The listing builds one solid part. Answer for the finished solid, in the listing's coordinates (mm). Face numbers are marked on the shaded views. A direction names the side the tool comes from. Round coordinates to 2 decimals unless told otherwise and drop trailing zeros. Order: outer loops, then holes, each group sorted by start corner. A loop starts at its lowest first (then second) coordinate and runs counter-clockwise, first axis right, second up. Notation, with made-up numbers: M 17,63 L 62,63 A17 cw 62,70 Z; hole C 74,59.25 d7. An arc over 180 degrees is marked long. Write item = value, one per line. Start each with the question number.
(1) A cutting plane is placed at C-C, the plane y = -41. Determine the outline of the cut face in (x, z).
(2) A cutting plane is placed at D-D, the plane x = -1. Determine the outline of the cut face in (y, z).
(3) For a pull along X with two mould halves and no side action, classify the marked faces 1, 2, 3 and 4 as released by +X, released by -X, zero draft, split by the parting line, or undercut.
(4) Straight lines are drawn through the part: probe 1 along X at (y, z) = (-48, 10.5); probe 2 along X at (y, z) = (-44, 1.5); probe 3 along Y at (x, z) = (19, 5). For each, find the intervals that lie inside material, in ascending order. Write a range as from..to.
(5) Which of the six approach directions +Z, -Z, +X, -X, +Y, -Y give full straight-line access (tool end or side, diameter ignored) to the marked faces 5, 6 and 7?
(6) Each of these flat-tipped pins is pushed along its axis until it touches: pin 1 (0.5 mm diameter, centred on y = -54.5, z = 10.5, fed in from -X); pin 2 (2.5 mm diameter, centred on x = -61.5, z = 6.5, fed in from +Y); pin 3 (6 mm diameter, centred on x = -56.5, z = 11, fed in from -Y). Where does it stop, or does it pass through?
(7) A cutting plane is placed at B-B, the plane x = -88. Determine the outline of the cut face in (y, z), and give its area (3 significant figures).
(8) A cutting plane is placed at A-A, the plane z = 9. Determine the outline of the cut face in (x, y).
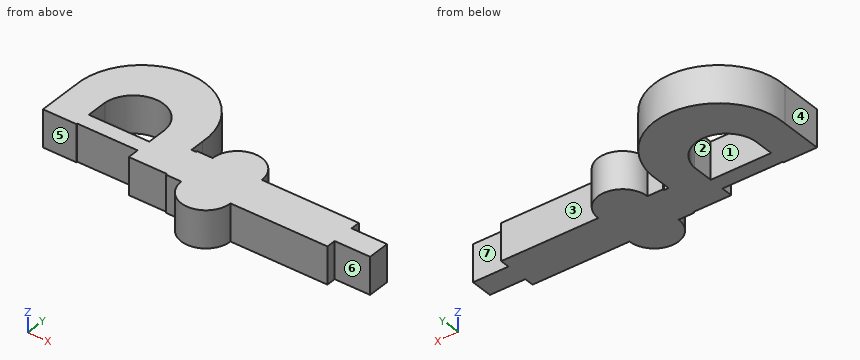
from build123d import *

# Parameters (mm, degrees)
F0_W     = 17
F0_H     = 10.514781
F1_DEPTH = 17.78


with BuildPart() as f1:
    # F0 (on Top) → F1 (new body)
    with BuildSketch(Plane.XY):
        with BuildLine():
            Line((-63.051145, -54.98954), (-63.051145, -48.261526))
            ThreePointArc((-63.051145, -48.261526), (-93.559145, -15.989189), (-124.067145, -48.261526))
            Line((-124.067145, -48.261526), (-124.067145, -54.989189))
            Line((-124.067145, -54.989189), (-124.067145, -56.005189))
            Line((-124.067145, -56.005189), (-124.067145, -68.254414))
            Line((-124.067145, -68.254414), (-108.051145, -68.254414))
            Line((-108.051145, -68.254414), (-108.051145, -67.754308))
            Line((-108.051145, -67.754308), (-108.051145, -60.490071))
            Line((-108.051145, -60.490071), (-108.051145, -56.005189))
            Line((-108.051145, -56.005189), (-108.051145, -54.989189))
            Line((-108.051145, -54.989189), (-108.051145, -50.514857))
            ThreePointArc((-108.051145, -50.514857), (-93.559145, -37.005189), (-79.067145, -50.514857))
            Line((-79.067145, -50.514857), (-79.067145, -54.98954))
            Line((-79.067145, -54.98954), (-63.051145, -54.98954))
        make_face()
        Polygon((-79.067145, -61.005189), (-79.067145, -60.490071), (-108.051145, -60.490071), (-108.051145, -67.754308), (-79.067145, -67.754308), align=None)
        Polygon((-60.801145, -54.98954), (-63.051145, -54.98954), (-79.067145, -54.98954), (-79.067145, -60.490071), (-79.067145, -61.005189), (-79.067145, -67.754308), (-79.067145, -73.254839), (-60.801145, -73.254839), align=None)
        Polygon((-60.801145, -54.364518), (-60.801145, -54.98954), (-60.801145, -73.254839), (-60.801145, -73.879861), (-53.390384, -73.879861), (-29.825188, -73.879861), (-23.928846, -73.879861), (16.698855, -73.879861), (16.698855, -69.37958), (16.698855, -58.864799), (16.698855, -54.364518), (-29.825188, -54.364518), (-53.390384, -54.364518), align=None)
        with Locations((25.198855, -64.122189)):
            Rectangle(F0_W, F0_H)
        with BuildLine():
            ThreePointArc((-29.825188, -54.364518), (-41.607786, -42.515753), (-53.390384, -54.364518))
            Line((-53.390384, -54.364518), (-29.825188, -54.364518))
        make_face()
        with BuildLine():
            Line((-29.825188, -73.879861), (-53.390384, -73.879861))
            ThreePointArc((-53.390384, -73.879861), (-41.607786, -85.662459), (-29.825188, -73.879861))
        make_face()
    extrude(amount=F1_DEPTH)


solid = f1.part
Reported:
q1.outline = M -123.61,0 L -103.56,0 L -103.56,17.78 L -123.61,17.78 Z; M -83.55,0 L -63.51,0 L -63.51,17.78 L -83.55,17.78 Z
q2.outline = M -73.88,0 L -54.36,0 L -54.36,17.78 L -73.88,17.78 Z
q3.face_1 = undercut
q3.face_2 = undercut
q3.face_3 = zero draft
q3.face_4 = released by -X
q4.probe_1 = -124.08..-107.65, -79.47..-63.04, -51.57..-31.65
q4.probe_2 = -124.01..-105.98, -81.14..-63.11, -47.33..-35.88
q4.probe_3 = -69.38..-58.86
q5.face_5 = +Z, -Z, -X, -Y
q5.face_6 = +Z, -Z, +X, -Y
q5.face_7 = +Z, -Z, +X, +Y
q6.pin_1 = -124.07
q6.pin_2 = -54.36
q6.pin_3 = -73.88
q7.outline = M -67.75,0 L -60.49,0 L -60.49,17.78 L -67.75,17.78 Z; M -38.11,0 L -16.5,0 L -16.5,17.78 L -38.11,17.78 Z
q7.area = 513 mm²
q8.outline = M -124.07,-68.25 L -108.05,-68.25 L -108.05,-67.75 L -79.07,-67.75 L -79.07,-73.25 L -60.8,-73.25 L -60.8,-73.88 L -53.39,-73.88 A11.78 ccw -29.83,-73.88 L 16.7,-73.88 L 16.7,-69.38 L 33.7,-69.38 L 33.7,-58.86 L 16.7,-58.86 L 16.7,-54.36 L -29.83,-54.36 A11.78 ccw long -53.39,-54.36 L -60.8,-54.36 L -60.8,-54.99 L -63.05,-54.99 L -63.05,-48.26 A30.56 ccw long -124.07,-48.26 Z; hole M -108.05,-60.49 L -79.07,-60.49 L -79.07,-50.51 A14.53 ccw -108.05,-50.51 Z
